Work out the finished part from the listing and answer in its coordinate system (mm). Coordinates: 2 decimals unless noted, no trailing zeros. Order: outer loops, then holes, each group sorted by start corner. A loop starts at its lowest first (then second) coordinate and runs counter-clockwise, first axis right, second up.
1. The part is cut by section B-B, the plane z = -132.5. Give the vertices of the cut face in (x, y).
2. Flat-ended cylindrical pins translate along their axes: pin 1 Ø1 at (x, z) = (-2.5, -95) entering from +Y; pin 2 Ø4.5 at (x, z) = (0.5, 10.5) entering from +Y. Find the tip coordinate at first contact, or state that the pin passes through.
3. The part is cut by section C-C, the plane y = -2.5. Give the vertices of the cut face in (x, z), then the cut area to 3 significant figures.
4. The part is cut by section A-A, the plane x = -1.75. Give the vertices of the cut face in (y, z), then the cut area to 3 significant figures.
5. Find the intervals of material crossed by probe 1 along Y at (x, z) = (-1, -38.5); probe 2 along Y at (x, z) = (6, 54); probe 3 along X at (y, z) = (3.5, -64.5), in increasing order.
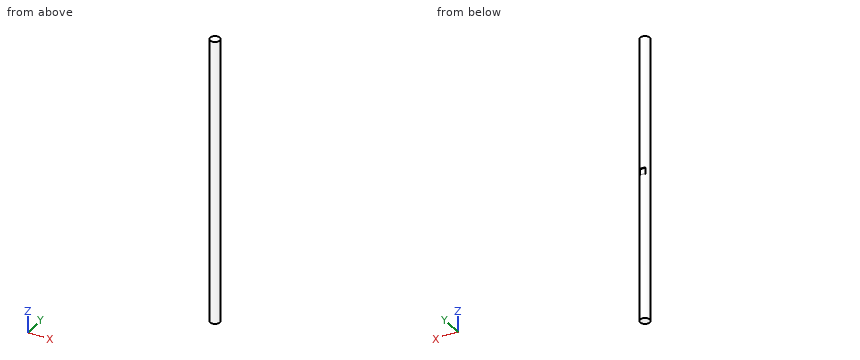
Autodesk Inventor part; units mm, degrees
ref_plane "Plano de trabajo1" through (0, 0, 5) normal (0, 0, 1) x (1, 0, 0)
ref_plane "YZ Plane" through (0, 0, 0) normal (1, 0, 0) x (0, 1, 0)
ref_plane "XZ Plane" through (0, 0, 0) normal (0, 1, 0) x (-1, 0, 0)
sketch "Boceto1" plane through (0, 0, 0) normal (0, 0, 1) x (1, 0, 0)
  circle A0 centre (0, 0) radius 7.5
  dimension "d0" = 15
extrude "Extrusión1" add sketch "Boceto1" along normal mid plane 450
ref_plane "Plano de trabajo1" through (0, 0, 5) normal (0, 0, 1) x (1, 0, 0)
sketch "Boceto5" plane through (0, 0, 5) normal (0, 0, 1) x (1, 0, 0)
  circle A0 centre (0, 0) radius 7.5
  circle A1 centre (0, 0) radius 7.5
  line L0 (0, 0) -> (0, 7.5)
  line L1 (0, 7.5) -> (0, 6)
  line L2 (0, 6) -> (4.5, 6)
  arc A2 (4.5, 6) -> (-4.5, 6) centre (0, 0) ccw
  line L3 (0, 6) -> (-4.5, 6)
  point P0 (-4.5, 6)
  dimension "d10" = 15
  dimension "d11" = 1.5
extrude "Extrusión4" cut sketch "Boceto5" along normal blind 10 contours L2 L0 A0 | A0 L0 L3
properties part number "Eje_Engranes_llanta"
Geometry says:
1. outline: circle Ø15 at (0, 0)
2. pin 1: stops at y = 7.23
2. pin 2: stops at y = 6
3. outline: (-7.07, -225) - (7.07, -225) - (7.07, 225) - (-7.07, 225) - close
3. area: 6,360 mm2
4. outline: (-7.29, -225) - (7.29, -225) - (7.29, 5) - (6, 5) - (6, 15) - (7.29, 15) - (7.29, 225) - (-7.29, 225) - close
4. area: 6,550 mm2
5. probe 1: y = -7.43 to 7.43
5. probe 2: y = -4.5 to 4.5
5. probe 3: x = -6.63 to 6.63
